Autodesk Inventor part; units mm, degrees
ref_plane "YZ Plane" through (0, 0, 0) normal (1, 0, 0) x (0, 1, 0)
ref_plane "XZ Plane" through (0, 0, 0) normal (0, 1, 0) x (-1, 0, 0)
ref_plane "XY Plane" through (0, 0, 0) normal (0, 0, 1) x (1, 0, 0)
sketch "Sketch1" plane through (0, 0, 0) normal (0, 0, 1) x (1, 0, 0)
  circle A0 centre (0, 0) radius 6.35
  dimension "d0" = 12.7
extrude "Extrusion1" add sketch "Sketch1" against normal blind 12.065
sketch "Sketch2" plane through (0, 0, 0) normal (0, 0, 1) x (1, 0, 0)
  circle A0 centre (0, 0) radius 6.35
  circle A1 centre (0, 0) radius 4.7625
  dimension "d3" = 9.525
extrude "Extrusion2" cut sketch "Sketch2" against normal blind 5.715
sketch "Sketch3" plane through (0, 0, 0) normal (0, 0, 1) x (1, 0, 0)
  circle A0 centre (0, 0) radius 4.7625
  circle A1 centre (0, 0) radius 2.4447
  dimension "d6" = 4.8895
extrude "Extrusion3" cut sketch "Sketch3" against normal through all contours A1
properties part number "T-Spacer .375"
Work out the finished part from the listing and answer in its coordinate system (mm). A direction names the side the tool comes from. Give positions to 0.01 mm unless a question says otherwise; leave off trailing zeros. Loops run counter-clockwise (first coordinate to the right, second up) from the corner with the lowest first, then second, coordinate; pieces in that order, holes last. Notation, with made-up numbers: (45.25, 76.5) -> (70.25, 76.5) arc R22 cw to (70.25, 86.5) -> close; hole circle Ø6 at (-11.5, 45). An arc over 180 degrees is marked (long way). Write item = value, one per line. Start each with the question number.
(1) Find section C-C on y = 3.5. Give the vertices of the cut face in (x, z) (3 decimals).
(2) The mould has two halves that part along X. Classify faces 3 (the cylindrical face through (-3.78, -2.9, -2.82)), 4 (the flat face through (3, 0, -12.065)), 5 (the cylindrical face through (2.332, 0.734, -5.948)): +X half, -X half, draft (parallel to the pull), parting line (faces both ways), or undercut.
(3) Given pin 1 Ø1 at (x, y) = (1, 1.5) entering from +Z; pin 2 Ø4 at (x, z) = (2.5, -10) entering from -Y; pin 3 Ø1.5 at (y, z) = (3.5, -6.5) entering from +X; pin 4 Ø1.5 at (x, z) = (-4.5, -9.5) entering from -Y, each flat-ended and moving along its own axis, determine where each tip first touches the part or whether it passes through.
(4) Which of the six approach directions +Z, -Z, +X, -X, +Y, -Y give full straight-line access (tool end or side, diameter ignored) to faces 1 (the flat face through (1, 5, -5.715)), 2 (the cylindrical face through (-1.38, -6.2, -8.85))?
(5) Find the intervals of material crossed by probe 1 along Y at (x, z) = (0, -5.5); probe 2 along Y at (x, z) = (0, -8); probe 3 along Z at (x, y) = (5.5, 0.5) (3 decimals), in increasing order. Write a range as from..to.
(6) Find section D-D on z = -1.5. Give the vertices of the cut face in (x, y) (1 decimal).
From the geometry:
q1.outline = (-5.298, -12.065) -> (5.298, -12.065) -> (5.298, -5.715) -> (3.23, -5.715) -> (3.23, 0) -> (-3.23, 0) -> (-3.23, -5.715) -> (-5.298, -5.715) -> close
q2.face_3 = parting line
q2.face_4 = draft
q2.face_5 = undercut
q3.pin_1 = through
q3.pin_2 = -6.33
q3.pin_3 = 5.72
q3.pin_4 = -5.12
q4.face_1 = +Z
q4.face_2 = +Z, -Z
q5.probe_1 = -4.76..-2.44, 2.44..4.76
q5.probe_2 = -6.35..-2.44, 2.44..6.35
q5.probe_3 = -12.065..-5.715
q6.outline = circle Ø9.5 at (0, 0); hole circle Ø4.9 at (0, 0)
